Could you check a few things on this model? Use its own coordinates, in mm. A direction names the side the tool comes from. Give positions to 0.01 mm unless a question says otherwise; leave off trailing zeros. Order: outer loops, then holes, each group sorted by start corner. A loop starts at its lowest first (then second) coordinate and runs counter-clockwise, first axis right, second up. Notation, with made-up numbers: (73.25, 68.25) - (123.25, 68.25) arc R10 ccw to (123.25, 84.25) - close; hole circle Ø8 at (69.5, 59). An arc over 180 degrees is marked (long way). Put each result on its own line as item: value.
from build123d import *

# Parameters (mm, degrees)
SKETCH1_R           = 46.5
SKETCH1_R_2         = 45.3
BOSS_EXTRUDE1_DEPTH = 40
SKETCH2_R           = 1.65
CUT_EXTRUDE1_DEPTH  = 77.970773674
CIRPATTERN1_COUNT   = 4
BOSS_EXTRUDE2_START = 2
SKETCH3_R           = 46.5
SKETCH3_R_2         = 41.5
BOSS_EXTRUDE2_DEPTH = 2


with BuildPart() as part:
    # Sketch1 → Boss-Extrude1 (new body)
    with BuildSketch(Plane(origin=(0, 0, 0), x_dir=(1, 0, 0), z_dir=(0, 1, 0))):
        with Locations(Location((0, 0, 0), (0, 0, 270))):
            Circle(SKETCH1_R)
        with Locations(Location((0, 0, 0), (0, 0, 270))):
            Circle(SKETCH1_R_2, mode=Mode.SUBTRACT)
    extrude(amount=BOSS_EXTRUDE1_DEPTH)

    # Sketch2 → Cut-Extrude1 (cut, through all)
    with BuildSketch(Plane(origin=(0, 0, 0), x_dir=(0, 0, -1), z_dir=(1, 0, 0))):
        with Locations((0, 35)):
            Circle(SKETCH2_R)
    cut_extrude1 = extrude(amount=-CUT_EXTRUDE1_DEPTH, mode=Mode.SUBTRACT)

    # CirPattern1: Cut-Extrude1 ×4 about axis
    cirpattern1_axis = Axis((0, 40, 0), (0, -1, 0))
    for i in range(1, CIRPATTERN1_COUNT):
        add(cut_extrude1.rotate(cirpattern1_axis, i * 360 / CIRPATTERN1_COUNT), mode=Mode.SUBTRACT)

    # Sketch3 → Boss-Extrude2 (add)
    with BuildSketch(Plane.XZ.offset(BOSS_EXTRUDE2_START)):
        with Locations(Location((0, 0, 0), (0, 0, 270))):
            Circle(SKETCH3_R)
        with Locations(Location((0, 0, 0), (0, 0, 270))):
            Circle(SKETCH3_R_2, mode=Mode.SUBTRACT)
    extrude(amount=-BOSS_EXTRUDE2_DEPTH)


solid = part.part
1) Suppose I cut it at A-A, the plane x = 0. List the corners of the cut face in (y, z) for me.
Filled in:
outline: (-2, -46.5) - (33.35, -46.5) - (33.35, -45.3) - (0, -45.3) - (0, -41.5) - (-2, -41.5) - close; (-2, 41.5) - (0, 41.5) - (0, 45.3) - (33.35, 45.3) - (33.35, 46.5) - (-2, 46.5) - close; (36.65, -46.5) - (40, -46.5) - (40, -45.3) - (36.65, -45.3) - close; (36.65, 45.3) - (40, 45.3) - (40, 46.5) - (36.65, 46.5) - close
2) Suppose I cut it at D-D, the plane z = -14. List the corners of the cut face in (x, y) for me.
Filled in:
outline: (-44.34, -2) - (-39.07, -2) - (-39.07, 0) - (-43.08, 0) - (-43.08, 40) - (-44.34, 40) - close; (39.07, -2) - (44.34, -2) - (44.34, 40) - (43.08, 40) - (43.08, 0) - (39.07, 0) - close
3) Which directions (+Z, -Z, +X, -X, +Y, -Y) give clear straight access to the entire face, cutting with the end or side of a thin tool? Please do faces 1 (the flat face through (-45, 40, 10)), 2 (the cylindrical face through (-27.56, 19.72, -35.95)).
Filled in:
face 1: +Z, -Z, +X, -X, +Y
face 2: +Y
4) I'm going to push flat-ended pins straight in: pin 1 (8 mm diameter, centred on y = 27, z = 36, fed in from +X); pin 2 (5.5 mm diameter, centred on y = 35, z = 0, fed in from -X); pin 3 (1 mm diameter, centred on x = -4.5, y = 18, fed in from +Z); pin 4 (3 mm diameter, centred on x = 19, y = 15, fed in from -Z). Where does each tip first touch, or does it pass through?
Filled in:
pin 1: stops at x = 33.74
pin 2: stops at x = -46.5
pin 3: stops at z = 46.33
pin 4: stops at z = -43.08
5) If I drill on line 1 (Z direction, x = 0, y = 17); line 2 (Z direction, x = -8, y = 25), over which ranges is the centre line in solid material (lowest first)? Write a range as [from, to].
Filled in:
line 1: z = [-46.5, -45.3], [45.3, 46.5]
line 2: z = [-45.81, -44.59], [44.59, 45.81]
6) Suppose I cut it at B-B, the plane z = 0. List the corners of the cut face in (x, y) for me.
Filled in:
outline: (-46.5, -2) - (-41.5, -2) - (-41.5, 0) - (-45.3, 0) - (-45.3, 33.35) - (-46.5, 33.35) - close; (-46.5, 36.65) - (-45.3, 36.65) - (-45.3, 40) - (-46.5, 40) - close; (41.5, -2) - (46.5, -2) - (46.5, 33.35) - (45.3, 33.35) - (45.3, 0) - (41.5, 0) - close; (45.3, 36.65) - (46.5, 36.65) - (46.5, 40) - (45.3, 40) - close
7) Suppose I cut it at C-C, the plane y = 35. List the corners of the cut face in (x, z) for me.
Filled in:
outline: (-46.47, -1.65) arc R46.5 ccw to (-1.65, -46.47) - (-1.65, -45.27) arc R45.3 cw to (-45.27, -1.65) - close; (-46.47, 1.65) - (-45.27, 1.65) arc R45.3 cw to (-1.65, 45.27) - (-1.65, 46.47) arc R46.5 ccw to start; (1.65, -46.47) arc R46.5 ccw to (46.47, -1.65) - (45.27, -1.65) arc R45.3 cw to (1.65, -45.27) - close; (1.65, 45.27) arc R45.3 cw to (45.27, 1.65) - (46.47, 1.65) arc R46.5 ccw to (1.65, 46.47) - close
8) We'd pull the mould along Y, two halves only. Please class faces 3 (the cylindrical face through (12.465, -1.014, -39.584)), 4 (the cylindrical face through (-45.88, 36.39, -0.89)), 5 (the flat face through (-37, 0, -20)): pulls with the +Y half, pulls with the -Y half, needs draft (parallel to the pull), parting line crosses it, or undercut.
Filled in:
face 3: needs draft
face 4: undercut
face 5: pulls with the +Y half
